Geometry check sheet. Reference: drawing and pictorial views, mm from the part's lowest x, y, z. A direction names the side the tool comes from. Coordinates: 2 decimals unless noted, no trailing zeros. Loops run counter-clockwise (first coordinate to the right, second up) from the corner with the lowest first, then second, coordinate; pieces in that order, holes last. Notation, with made-up numbers: (80, 49.5) -> (106, 49.5) arc R19 ccw to (106, 56.5) -> close; hole circle Ø5 at (24.25, -2.75). An arc over 180 degrees is marked (long way). Use one line per item in the form item = value.
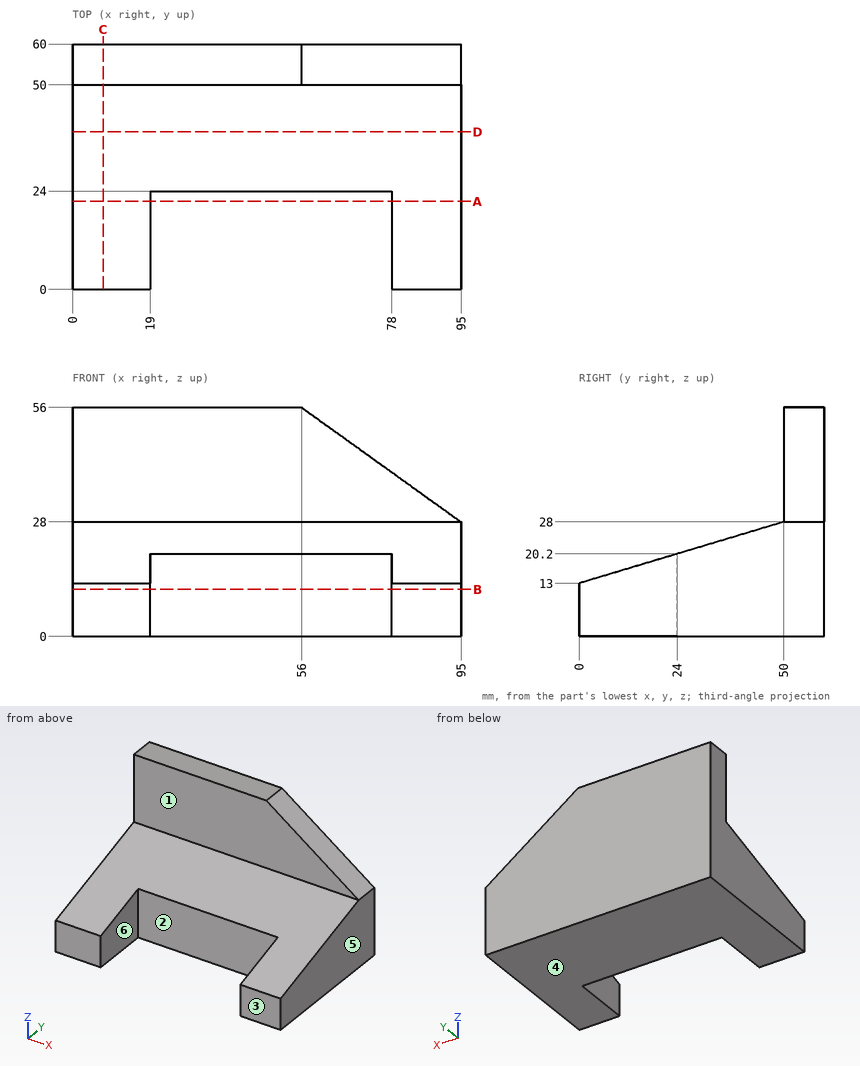
(1) Section check D-D, the plane y = 38.5. Record the boundary of the cut face in (x, z), plus the area to 3 significant figures.
Established:
outline = (0, 0) -> (95, 0) -> (95, 24.55) -> (0, 24.55) -> close
area = 2,330 mm²
(2) Section check A-A, the plane y = 21.5. Record the boundary of the cut face in (x, z).
Established:
outline = (0, 0) -> (19, 0) -> (19, 19.45) -> (0, 19.45) -> close; (78, 0) -> (95, 0) -> (95, 19.45) -> (78, 19.45) -> close
(3) Scan lines: line 1 along X through (y, z) = (6, 6); line 2 along Z through (x, y) = (82, 20); line 3 along Y through (x, z) = (9, 30). Record each from-to range of solid material in increasing order.
Established:
line_1 = 0 to 19, 78 to 95
line_2 = 0 to 19
line_3 = 50 to 60
(4) Tool access check on the marked faces 1, 2 and 3. Record the directions out of +Z, -Z, +X, -X, +Y, -Y that give a thin tool (end or side, any length) a straight path to the whole face; none if there is none.
Established:
face_1 = +Z, +X, -X, -Y
face_2 = +Z, -Z, -Y
face_3 = +Z, -Z, +X, -X, -Y
(5) Section check C-C, the plane x = 7.5. Record the boundary of the cut face in (y, z), plus the area to 4 significant figures.
Established:
outline = (0, 0) -> (60, 0) -> (60, 56) -> (50, 56) -> (50, 28) -> (0, 13) -> close
area = 1,585 mm²
(6) Mould release check, pull along X, two halves, no side actions. Record for the marked faces 4, 5 and 6: +X half, -X half, draft (parallel to the pull), parting line (faces both ways), or undercut.
Established:
face_4 = draft
face_5 = +X half
face_6 = undercut
(7) Section check B-B, the plane z = 11.5. Record the boundary of the cut face in (x, y), plus the area to 3 significant figures.
Established:
outline = (0, 0) -> (19, 0) -> (19, 24) -> (78, 24) -> (78, 0) -> (95, 0) -> (95, 60) -> (0, 60) -> close
area = 4,280 mm²
(8) Go/stop test with flat-tipped pins: P1, Ø16, axis at x = 41.5, z = 12, coming from the -Y side; P2, Ø22.5, axis at x = 70, z = 46.5, coming from the -Y side; P3, Ø6, axis at x = 52.5, y = 37, coming from the +Z side. Record where each tip stops, or that it passes through.
Established:
P1 = 24
P2 = 50
P3 = 25
